```python
from build123d import *

# Parameters (mm, degrees)
F0_R     = 7.1
F1_DEPTH = 14
F2_R     = 8.5
F2_R_2   = 7.1
F3_DEPTH = 3
F4_R     = 2.99999
F5_W     = 17
F5_H     = 17
F5_R     = 7.1
F6_DEPTH = 3


# Not quite as in the source:
# - a fillet or chamfer is up to 0.001 mm smaller than in the source, because OpenCascade refuses the exact size


with BuildPart() as f1:
    # F0 (on Front) → F1 (new body)
    with BuildSketch(Plane.XZ):
        Circle(F0_R)
    extrude(amount=F1_DEPTH)

    # F2 (on face) → F3 (join)
    with BuildSketch(Plane.XZ.offset(14)):
        Circle(F2_R)
        Circle(F2_R_2, mode=Mode.SUBTRACT)
        Circle(F2_R_2)
    extrude(amount=F3_DEPTH)

    # F4 (radius 3 in the source; OpenCascade refuses exactly that, so slightly less here)
    f4_edges = [f1.edges().sort_by_distance(p)[0] for p in [
        (-8.5, -17, 0),
    ]]
    fillet(f4_edges, radius=F4_R)

    # F5 (on face) → F6 (join)
    with BuildSketch(Plane(origin=(0, 0, 0), x_dir=(-1, 0, 0), z_dir=(0, 1, 0))):
        with Locations((2.794e-06, 0)):
            Rectangle(F5_W, F5_H)
        Circle(F5_R, mode=Mode.SUBTRACT)
        Circle(F5_R)
    extrude(amount=F6_DEPTH)


solid = f1.part
```
Can you work these out from the model? Positions are in its coordinate system, mm. A direction names the side the tool comes from. Give positions to 0.01 mm unless a question says otherwise; leave off trailing zeros. Order: outer loops, then holes, each group sorted by start corner. A loop starts at its lowest first (then second) coordinate and runs counter-clockwise, first axis right, second up. Notation, with made-up numbers: (39.5, -16.75) - (96.5, -16.75) arc R25 ccw to (96.5, 20.25) - close; hole circle Ø1 at (13.25, -3.75). An arc over 180 degrees is marked (long way). Use a Markdown table: item, result. Add a question column.
Q1. Please list where these lines run through material, in increasing order: line 1 along Y through (x, z) = (5.75, -7); line 2 along X through (y, z) = (-9.75, -6.5); line 3 along Z through (x, y) = (0.75, -11.25).
Q2. If we mould it in two halves opening along Y, with no side actions, what happens to faces 1 (the flat face through (0, 1, 8.5)), 2 (the flat face through (8, 0, 0)), 3 (the flat face through (0, -17, 0))? For each: released by +Y, released by -Y, zero draft, split by the parting line, or undercut.
Q3. If we section it at C-C on y = -12.5: Write out the boundary of the cut face in (x, z), plus the area to 3 significant figures.
Q4. I'm going to push flat-ended pins straight in: pin 1 (5 mm diameter, centred on y = -10, z = 1.5, fed in from -X); pin 2 (1.5 mm diameter, centred on y = -11, z = -2, fed in from -X); pin 3 (1 mm diameter, centred on x = 2.5, y = -13, fed in from -Z). Where does each tip first touch, or does it pass through?
Q5. On a 3-axis mill with a long thin cutter (end or side, diameter ignored), from which of +Z, -Z, +X, -X, +Y, -Y can I reach the whole of each face in a straight line? I mean faces 4 (the flat face through (-2, -14, -7)), 5 (the flat face through (8.5, 1, 0)). Say none if no direction works.
Answers follow:
| question | item | result |
|---|---|---|
| 1 | line 1 | y = 0 to 3 |
| 1 | line 2 | x = -2.86 to 2.86 |
| 1 | line 3 | z = -7.06 to 7.06 |
| 2 | face 1 | zero draft |
| 2 | face 2 | undercut |
| 2 | face 3 | released by -Y |
| 3 | outline | circle Ø14.2 at (0, 0) |
| 3 | area | 158 mm^2 |
| 4 | pin 1 | stops at x = -7.1 |
| 4 | pin 2 | stops at x = -6.99 |
| 4 | pin 3 | stops at z = -6.81 |
| 5 | face 4 | none |
| 5 | face 5 | +Z, -Z, +X, +Y, -Y |
